Geometry check sheet. Reference: the model listing, model coordinates, mm. A direction names the side the tool comes from. Round coordinates to 2 decimals unless told otherwise and drop trailing zeros. Order: outer loops, then holes, each group sorted by start corner. A loop starts at its lowest first (then second) coordinate and runs counter-clockwise, first axis right, second up. Notation, with made-up numbers: (23.5, -33) -> (46.5, -33) arc R16 cw to (46.5, -14) -> close; hole circle Ø11 at (-17.5, 86). An arc over 180 degrees is marked (long way). Use a Markdown table: item, result. Add a question column.
Item 1: Sectioned sample at B-B, the plane y = -15. Record the cut outline in (x, z), and give its area (3 significant figures).
Item 2: Set-up check for faces 4 (the cylindrical face through (5, -13, 1)), 5 (the flat face through (-20, -63, 20)), 6 (the flat face through (-10, -62, 26)): record each of +Z, -Z, +X, -X, +Y, -Y from which the full face is reachable in a straight line by a thin tool's end or side.
Item 3: Sectioned sample at A-A, the plane x = -5. Record the cut outline in (y, z).
Item 4: Gauge pin test, flat ends, axial feed: pin 1 Ø13.5 at (y, z) = (-26, 9.5) entering from -X; pin 2 Ø3.5 at (x, y) = (-23.5, -63) entering from -Z; pin 3 Ø4 at (x, y) = (-10.5, -43.5) entering from +Z. Record the tip position at first contact, or that the pin passes through.
Item 5: Sectioned sample at C-C, the plane x = 1. Record the cut outline in (y, z).
Item 6: Mould release check, pull along Y, two halves, no side actions. Record for faces 1 (the cylindrical face through (-5, -13, 1)), 2 (the flat face through (0, 0, 1)), 3 (the flat face through (10, -42, 2)): pulls with the +Y half, pulls with the -Y half, needs draft (parallel to the pull), parting line crosses it, or undercut.
Item 7: Material ranges on probe 1 along Y at (x, z) = (-6, 32.5); probe 2 along Y at (x, z) = (-5, 1); probe 3 along Y at (x, z) = (5, 2.35), recorded low to high. Write a range as [from, to].
Item 8: Sectioned sample at D-D, the plane z = 30. Record the cut outline in (x, y), and give its area (3 significant figures).
from build123d import *

# Parameters (mm, degrees)
SKETCH_1_W          = 20
SKETCH_1_H          = 65
SKETCH_1_R          = 2
EXTRUDE_1_DEPTH     = 3
SKETCH_2_W          = 40
SKETCH_2_H          = 3
EXTRUDE_2_DEPTH     = 40
SKETCH_3_W          = 20
SKETCH_3_H          = 20
CUT_EXTRUDE_1_DEPTH = 3
FILLET_1_R          = 10
FILLET_2_R          = 3


with BuildPart() as part:
    # 草图1 → 凸台-拉伸1 (new body)
    with BuildSketch(Plane.XY):
        with Locations((0, -32.5)):
            Rectangle(SKETCH_1_W, SKETCH_1_H)
        with Locations((-5, -15)):
            Circle(SKETCH_1_R, mode=Mode.SUBTRACT)
        with Locations((5, -15)):
            Circle(SKETCH_1_R, mode=Mode.SUBTRACT)
    extrude(amount=EXTRUDE_1_DEPTH)

    # 草图2 → 凸台-拉伸2 (add)
    with BuildSketch(Plane.XY):
        with Locations((-10, -63.5)):
            Rectangle(SKETCH_2_W, SKETCH_2_H)
    extrude(amount=EXTRUDE_2_DEPTH)

    # 草图3 → 切除-拉伸1 (cut)
    with BuildSketch(Plane(origin=(0, -62, 0), x_dir=(1, 0, 0), z_dir=(0, 1, 0))):
        with Locations((-20, -10)):
            Rectangle(SKETCH_3_W, SKETCH_3_H)
    extrude(amount=-CUT_EXTRUDE_1_DEPTH, mode=Mode.SUBTRACT)

    # 圆角1
    fillet_1_edges = [part.edges().sort_by_distance(p)[0] for p in [
        (0, -62, 3),
        (0, -65, 0),
    ]]
    fillet(fillet_1_edges, radius=FILLET_1_R)

    # 圆角2
    fillet_2_edges = [part.edges().sort_by_distance(p)[0] for p in [
        (-30, -63.5, 40),
        (10, -63.5, 40),
        (-30, -63.5, 20),
        (-10, -63.5, 20),
    ]]
    fillet(fillet_2_edges, radius=FILLET_2_R)


solid = part.part
Found:
| question | item | result |
|---|---|---|
| 1 | outline | (-10, 0) -> (-7, 0) -> (-7, 3) -> (-10, 3) -> close; (-3, 0) -> (3, 0) -> (3, 3) -> (-3, 3) -> close; (7, 0) -> (10, 0) -> (10, 3) -> (7, 3) -> close |
| 1 | area | 36.0 mm2 |
| 2 | face 4 | +Z, -Z |
| 2 | face 5 | -Z, -X, +Y, -Y |
| 2 | face 6 | +Z, +X, -X, +Y |
| 3 | outline | (-65, 10) arc R10 ccw to (-55, 0) -> (-17, 0) -> (-17, 3) -> (-52, 3) arc R10 cw to (-62, 13) -> (-62, 40) -> (-65, 40) -> close; (-13, 0) -> (0, 0) -> (0, 3) -> (-13, 3) -> close |
| 4 | pin 1 | stops at x = -10 |
| 4 | pin 2 | stops at z = 20 |
| 4 | pin 3 | stops at z = 3 |
| 5 | outline | (-65, 10) arc R10 ccw to (-55, 0) -> (0, 0) -> (0, 3) -> (-52, 3) arc R10 cw to (-62, 13) -> (-62, 40) -> (-65, 40) -> close |
| 6 | face 1 | undercut |
| 6 | face 2 | pulls with the +Y half |
| 6 | face 3 | needs draft |
| 7 | probe 1 | y = [-65, -62] |
| 7 | probe 2 | y = [-59.36, -17], [-13, 0] |
| 7 | probe 3 | y = [-61.44, -17], [-13, 0] |
| 8 | outline | (-30, -65) -> (10, -65) -> (10, -62) -> (-30, -62) -> close |
| 8 | area | 120 mm2 |
